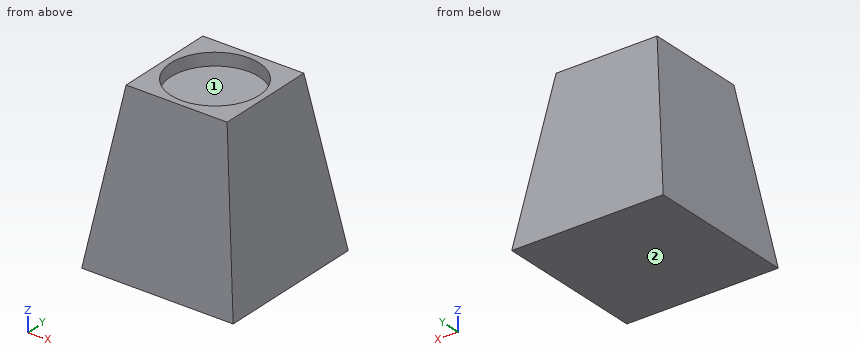
```python
from build123d import *

# Parameters (mm, degrees)
F0_W     = 120
F0_H     = 120
F2_W     = 80
F2_H     = 80
F4_R     = 35
F5_DEPTH = 10


with BuildPart() as f3:
    # F0 (on Top) → F3 section 0
    with BuildSketch(Plane.XY):
        Rectangle(F0_W, F0_H)
    # F2 (on offset) → F3 section 1
    with BuildSketch(Plane.XY.offset(130)):
        Rectangle(F2_W, F2_H)
    loft()

    # F4 (on face) → F5 (cut)
    with BuildSketch(Plane.XY.offset(130)):
        Circle(F4_R)
    extrude(amount=-F5_DEPTH, mode=Mode.SUBTRACT)


solid = f3.part
```
CAD build for the part. Positions are in the model's coordinates, mm. Face numbers are marked on the shaded views. Coordinates: 2 decimals unless noted, no trailing zeros. Write each question's results on one line, items separated by ' | '. Start each with the question number.
Q1. Pull direction Y, two halves, no side cores. Call the marked faces 1 and 2: +Y half, -Y half, draft (parallel to the pull), parting line (faces both ways), or undercut.
Q2. Drill centre lines: probe 1 along Z at (x, y) = (-26, -17.5); probe 2 along Y at (x, z) = (0, 126); probe 3 along Y at (x, z) = (0, 126.75). Where is each one in solid material? Low to high. Write a range as from..to.
Q3. Flat gauge pins, fed straight in: P1, Ø12, axis at y = -41.5, z = 98, coming from the +X side; P2, Ø2, axis at x = 43, z = 15, coming from the +Y side; P3, Ø1.5, axis at y = -7.5, z = 87.5, coming from the +X side. Where does each tip first touch, or does it go through?
Found:
1) face 1: undercut | face 2: draft
2) probe 1: 0..120 | probe 2: -40.62..-35, 35..40.62 | probe 3: -40.5..-35, 35..40.5
3) P1: x = 45.85 | P2: y = 57.85 | P3: x = 46.65
